```python
from build123d import *

# Parameters (mm, degrees)
SKETCH1_W                     = 520
SKETCH1_H                     = 234
BOSS_EXTRUDE1_DEPTH           = 10
SKETCH8_W                     = 20
SKETCH8_H                     = 8
CUT_EXTRUDE5_DEPTH            = 6
FILLET2_R                     = 2.5
CUT_EXTRUDE7_DEPTH            = 571.312195205
M4X0_7_TAPPED_HOLE1_D         = 3.3
M4X0_7_TAPPED_HOLE1_DEPTH     = 12
M4X0_7_TAPPED_HOLE1_TIP       = 0.991420021
CBORE_FOR_M4_SHCS1_AT_2_COUNT = 2
CBORE_FOR_M4_SHCS1_AT_2_PITCH = 70.5
CBORE_FOR_M4_SHCS1_AT_3_COUNT = 2
CBORE_FOR_M4_SHCS1_AT_3_PITCH = 141
M4X0_7_TAPPED_HOLE2_D         = 3.3
SKETCH18_R                    = 11.15
CUT_EXTRUDE8_DEPTH            = 571.312195205
SKETCH19_W                    = 35
SKETCH19_H                    = 47
CUT_EXTRUDE9_DEPTH            = 7
FILLET3_R                     = 2
CUT_EXTRUDE10_DEPTH           = 571.312195205
SKETCH21_R                    = 12.5
CUT_EXTRUDE11_DEPTH           = 7


with BuildPart() as part:
    # Sketch1 → Boss-Extrude1 (new body)
    with BuildSketch(Plane.XY):
        with Locations((260, 117)):
            Rectangle(SKETCH1_W, SKETCH1_H)
    extrude(amount=BOSS_EXTRUDE1_DEPTH)

    # Sketch8 → Cut-Extrude5 (cut)
    with BuildSketch(Plane.XY.offset(10)):
        with Locations((260, 232)):
            Rectangle(SKETCH8_W, SKETCH8_H)
    extrude(amount=-CUT_EXTRUDE5_DEPTH, mode=Mode.SUBTRACT)

    # Fillet2
    fillet2_edges = [part.edges().sort_by_distance(p)[0] for p in [
        (270, 231, 4),
        (250, 231, 4),
    ]]
    fillet(fillet2_edges, radius=FILLET2_R)

    # Sketch9 → Cut-Extrude7 (cut, through all)
    with BuildSketch(Plane(origin=(0, 0, 0), x_dir=(0, 0, -1), z_dir=(1, 0, 0))):
        Polygon((0, 234), (-10, 232.685250563), (-10, 234), align=None)
    extrude(amount=CUT_EXTRUDE7_DEPTH, mode=Mode.SUBTRACT)

    # M4x0.7 Tapped Hole1
    with Locations(Plane(origin=(0, 0, 0), x_dir=(-1, 0, 0), z_dir=(0, -1, 0))):
        with Locations((-70, -5), (-260, -5), (-450, -5)):
            Hole(M4X0_7_TAPPED_HOLE1_D / 2, depth=M4X0_7_TAPPED_HOLE1_DEPTH)
            with Locations((0, 0, -(M4X0_7_TAPPED_HOLE1_DEPTH + M4X0_7_TAPPED_HOLE1_TIP / 2))):  # 118° drill point
                Cone(0, M4X0_7_TAPPED_HOLE1_D / 2, M4X0_7_TAPPED_HOLE1_TIP, mode=Mode.SUBTRACT)

    # Sketch13 → CBORE for M4 SHCS1 (revolve, cut)
    with BuildSketch(Plane(origin=(5, 211.5, 10), x_dir=(0, -1, 0), z_dir=(1, 0, 0))):
        Polygon((0, 0), (0, 13.351936393), (2.25, 12), (2.25, 4), (4, 4), (4, 0), align=None)
    cbore_for_m4_shcs1 = revolve(axis=Axis((5, 211.5, 16.35), (0, 0, -1)), mode=Mode.SUBTRACT)

    # CBORE for M4 SHCS1 at 2: CBORE for M4 SHCS1 ×2
    with Locations(*[(0, -i * CBORE_FOR_M4_SHCS1_AT_2_PITCH, 0) for i in range(1, CBORE_FOR_M4_SHCS1_AT_2_COUNT)]):
        add(cbore_for_m4_shcs1, mode=Mode.SUBTRACT)

    # CBORE for M4 SHCS1 at 3: CBORE for M4 SHCS1 ×2
    with Locations(*[(0, -i * CBORE_FOR_M4_SHCS1_AT_3_PITCH, 0) for i in range(1, CBORE_FOR_M4_SHCS1_AT_3_COUNT)]):
        add(cbore_for_m4_shcs1, mode=Mode.SUBTRACT)

    # Mirror1: CBORE for M4 SHCS1 across plane
    add(cbore_for_m4_shcs1.mirror(Plane.ZY.offset(-260)), mode=Mode.SUBTRACT)

    # Mirror1 copy 1 sketch → Mirror1 copy 1 (revolve, cut)
    with BuildSketch(Plane(origin=(515, 141, 10), x_dir=(0, -1, 0), z_dir=(-1, 0, 0))):
        Polygon((0, 0), (0, -13.351936393), (2.25, -12), (2.25, -4), (4, -4), (4, 0), align=None)
    revolve(axis=Axis((515, 141, 16.35), (0, 0, 1)), mode=Mode.SUBTRACT)

    # Mirror1 copy 2 sketch → Mirror1 copy 2 (revolve, cut)
    with BuildSketch(Plane(origin=(515, 70.5, 10), x_dir=(0, -1, 0), z_dir=(-1, 0, 0))):
        Polygon((0, 0), (0, -13.351936393), (2.25, -12), (2.25, -4), (4, -4), (4, 0), align=None)
    revolve(axis=Axis((515, 70.5, 16.35), (0, 0, 1)), mode=Mode.SUBTRACT)

    # M4x0.7 Tapped Hole2 (through all)
    with Locations(Plane.XY.offset(10)):
        with Locations((116.15, 207.185250563), (116.15, 191.685250563)):
            m4x0_7_tapped_hole2 = Hole(M4X0_7_TAPPED_HOLE2_D / 2)

    # Mirror2: M4x0.7 Tapped Hole2 across plane
    add(m4x0_7_tapped_hole2.mirror(Plane.ZY.offset(-260)), mode=Mode.SUBTRACT)

    # Sketch17 → Ø9.0 (9) Diameter Hole1 (revolve, cut)
    with BuildSketch(Plane(origin=(116.15, 233.348234248, 4.957338137), x_dir=(0, -0.1303531504610662, 0.9914676273912701), z_dir=(1, 0, 0))):
        Polygon((0, 0), (0, 5.703872786), (4.5, 3), (4.5, 0), align=None)
    f_9_0_9_diameter_hole1 = revolve(axis=Axis((116.15, 239.644053682, 5.785080642), (0, -0.9914676273912703, -0.13035315046106621)), mode=Mode.SUBTRACT)

    # Mirror5: Ø9.0 (9) Diameter Hole1 across plane
    add(f_9_0_9_diameter_hole1.mirror(Plane.ZY.offset(-260)), mode=Mode.SUBTRACT)

    # Sketch18 → Cut-Extrude8 (cut, through all)
    with BuildSketch(Plane.XY.offset(10)):
        with Locations((260, 100)):
            Circle(SKETCH18_R)
    extrude(amount=-CUT_EXTRUDE8_DEPTH, mode=Mode.SUBTRACT)

    # Sketch19 → Cut-Extrude9 (cut)
    with BuildSketch(Plane(origin=(0, 0, 0), x_dir=(-1, 0, 0), z_dir=(0, 0, -1))):
        with Locations((-260, 106.5)):
            Rectangle(SKETCH19_W, SKETCH19_H)
    extrude(amount=-CUT_EXTRUDE9_DEPTH, mode=Mode.SUBTRACT)

    # Fillet3
    fillet3_edges = [part.edges().sort_by_distance(p)[0] for p in [
        (277.5, 83, 3.5),
        (277.5, 130, 3.5),
        (242.5, 130, 3.5),
        (242.5, 83, 3.5),
    ]]
    fillet(fillet3_edges, radius=FILLET3_R)

    # Sketch20 → Cut-Extrude10 (cut, through all)
    with BuildSketch(Plane(origin=(0, 0, 0), x_dir=(-1, 0, 0), z_dir=(0, 0, -1))):
        with BuildLine():
            Line((-75.5, 177.248182419), (-75.5, 182.751817581))
            ThreePointArc((-75.5, 182.751817581), (-63.85, 180), (-75.5, 177.248182419))
        make_face()
    cut_extrude10 = extrude(amount=-CUT_EXTRUDE10_DEPTH, mode=Mode.SUBTRACT)

    # Mirror6: Cut-Extrude10 across plane
    add(cut_extrude10.mirror(Plane.ZY.offset(-260)), mode=Mode.SUBTRACT)

    # Sketch21 → Cut-Extrude11 (cut)
    with BuildSketch(Plane(origin=(0, 0, 0), x_dir=(-1, 0, 0), z_dir=(0, 0, -1))):
        with Locations((-70, 180)):
            Circle(SKETCH21_R)
    cut_extrude11 = extrude(amount=-CUT_EXTRUDE11_DEPTH, mode=Mode.SUBTRACT)

    # Mirror7: Cut-Extrude11 across plane
    add(cut_extrude11.mirror(Plane.ZY.offset(-260)), mode=Mode.SUBTRACT)


solid = part.part
```
Input: part model. Units: mm. Frame: model coordinates. A direction names the side the tool comes from. Coordinates: 2 decimals unless noted, no trailing zeros. Loops run counter-clockwise (first coordinate to the right, second up) from the corner with the lowest first, then second, coordinate; pieces in that order, holes last.
Q1. Section A-A, the plane y = 100. Return the cut outline in (x, z), and give its area (3 significant figures).
Results are:
outline: (0, 0) - (242.5, 0) - (242.5, 7) - (248.85, 7) - (248.85, 10) - (0, 10) - close; (271.15, 7) - (277.5, 7) - (277.5, 0) - (520, 0) - (520, 10) - (271.15, 10) - close
area: 4,890 mm2
Q2. Contact query for flat-ended pins moving along their axis: pin 1 (6.5 mm diameter, centred on x = 515, y = 70.5, fed in from -Z); pin 2 (4.5 mm diameter, centred on x = 263, y = 231.5, fed in from +Z); pin 3 (1.5 mm diameter, centred on x = 183.5, z = 7.5, fed in from +Y); pin 4 (6 mm diameter, centred on x = 5, y = 70.5, fed in from +Z). Output: stop coordinate, or through.
Results are:
pin 1: stops at z = 0
pin 2: stops at z = 4
pin 3: stops at y = 233.11
pin 4: stops at z = 6
Q3. Set-up query: faces 5 (the flat face through (444, 180, 7)), 6 (the flat face through (0, 115, 5)). Return all of +Z, -Z, +X, -X, +Y, -Y with unobstructed straight access to the full face (end or side cutting, diameter ignored); none if empty.
Results are:
face 5: -Z
face 6: +Z, -Z, -X, +Y, -Y
Q4. Line query: line 1 along X through (y, z) = (70.5, 3.9); line 2 along X through (y, z) = (211.5, 7.5); line 3 along X through (y, z) = (90.5, 3). Output: solid intervals per line, ascending.
Results are:
line 1: x = 0 to 2.75, 7.25 to 512.75, 517.25 to 520
line 2: x = 0 to 1, 9 to 511, 519 to 520
line 3: x = 0 to 242.5, 277.5 to 520
Q5. Mould query, pull axis Z, two halves, no side actions, for faces 1 (the cylindrical face through (251.15, 93.22, 8.52)), 2 (the cylindrical face through (399.457, 232.009, 3.797)), 3 (the flat face through (260, 112, 7)), 4 (the flat face through (256.4, 233.5, 3.8)). Classes: +Z half, -Z half, draft (parallel to the pull), parting line (faces both ways), or undercut.
Results are:
face 1: draft
face 2: undercut
face 3: -Z half
face 4: +Z half
